```python
from build123d import *

# Parameters (mm, degrees)
SKETCH1_R           = 10.5
BOSS_EXTRUDE1_DEPTH = 10
SKETCH2_W           = 10.583005244
SKETCH2_H           = 12
BOSS_EXTRUDE2_DEPTH = 16
CUT_EXTRUDE1_REACH  = 34.181
SKETCH3_R           = 3
SKETCH4_R           = 8.7
BOSS_EXTRUDE3_DEPTH = 242
BOSS_EXTRUDE4_START = 10
SKETCH5_R           = 10.5
BOSS_EXTRUDE4_DEPTH = 10
BOSS_EXTRUDE5_START = 17
SKETCH6_R           = 8
BOSS_EXTRUDE5_DEPTH = 17
SKETCH7_R           = 3
CUT_EXTRUDE2_DEPTH  = 201


with BuildPart() as part:
    # Sketch1 → Boss-Extrude1 (new body)
    with BuildSketch(Plane.XY):
        Circle(SKETCH1_R)
    extrude(amount=BOSS_EXTRUDE1_DEPTH)

    # Sketch2 → Boss-Extrude2 (add)
    with BuildSketch(Plane.XY.offset(10)):
        Rectangle(SKETCH2_W, SKETCH2_H)
        with BuildLine():
            ThreePointArc((5.291502622, 6), (0, 8), (-5.291502622, 6))
            Line((-5.291502622, 6), (5.291502622, 6))
        make_face()
        with BuildLine():
            Line((5.291502622, -6), (-5.291502622, -6))
            ThreePointArc((-5.291502622, -6), (0, -8), (5.291502622, -6))
        make_face()
    extrude(amount=BOSS_EXTRUDE2_DEPTH)

    # Sketch3 → Cut-Extrude1 (cut, up to next)
    with BuildSketch(Plane(origin=(5.291502622, 0, 0), x_dir=(0, 0, -1), z_dir=(1, 0, 0)), mode=Mode.PRIVATE) as cut_extrude1_sk1:
        with Locations((-19, 0)):
            Circle(SKETCH3_R)
    cut_extrude1_tool1 = extrude(cut_extrude1_sk1.sketch, amount=-CUT_EXTRUDE1_REACH, mode=Mode.PRIVATE) & part.part
    add(cut_extrude1_tool1.solids().sort_by_distance((5.291503, 0, 19))[0], mode=Mode.SUBTRACT)

    # Sketch4 → Boss-Extrude3 (add)
    with BuildSketch(Plane(origin=(0, 0, 0), x_dir=(-1, 0, 0), z_dir=(0, 0, -1))):
        with Locations(Location((0, 0, 0), (0, 0, 180))):
            Circle(SKETCH4_R)
    extrude(amount=BOSS_EXTRUDE3_DEPTH)

    # Sketch5 → Boss-Extrude4 (add)
    with BuildSketch(Plane(origin=(0, 0, -242), x_dir=(-1, 0, 0), z_dir=(0, 0, -1)).offset(BOSS_EXTRUDE4_START)):
        with Locations(Location((0, 0, 0), (0, 0, 180))):
            Circle(SKETCH5_R)
    extrude(amount=-BOSS_EXTRUDE4_DEPTH)

    # Sketch6 → Boss-Extrude5 (add)
    with BuildSketch(Plane(origin=(0, 0, -252), x_dir=(-1, 0, 0), z_dir=(0, 0, -1)).offset(BOSS_EXTRUDE5_START)):
        Circle(SKETCH6_R)
    extrude(amount=-BOSS_EXTRUDE5_DEPTH)

    # Sketch7 → Cut-Extrude2 (cut)
    with BuildSketch(Plane(origin=(0, 0, -269), x_dir=(-1, 0, 0), z_dir=(0, 0, -1))):
        Circle(SKETCH7_R)
    extrude(amount=-CUT_EXTRUDE2_DEPTH, mode=Mode.SUBTRACT)


solid = part.part
```
Check sheet for the modelled part. Datum: model origin and axes. Units: mm. A direction names the side the tool comes from. Give positions to 0.01 mm unless a question says otherwise; leave off trailing zeros. Order: outer loops, then holes, each group sorted by start corner. A loop starts at its lowest first (then second) coordinate and runs counter-clockwise, first axis right, second up. Notation, with made-up numbers: M 33,21.5 L 72,21.5 A31 cw 72,57.5 Z; hole C -36.75,87 d3. An arc over 180 degrees is marked long. Answer in a Markdown table with one row per item.
1) Thickness scan on L1, parallel to Y at x = 0, z = -216.5; L2, parallel to Z at x = -8, y = -6.75; L3, parallel to Z at x = 2, y = -0.25. Record the ranges inside material, lowest first. Write a range as [from, to].
Filled sheet:
| item | result |
|---|---|
| L1 | y = [-8.7, -3], [3, 8.7] |
| L2 | z = [-252, -242], [0, 10] |
| L3 | z = [-68, 16.01], [21.99, 26] |
2) Gauge pin test, flat ends, axial feed: P1, Ø1.5, axis at x = 5.5, z = -48.5, coming from the +Y side; P2, Ø12, axis at x = 5, z = -136.5, coming from the -Y side; P3, Ø3.5, axis at y = -1, z = 17, coming from the +X side; P4, Ø10, axis at x = 6, y = 1, coming from the +Z side. Record the tip position at first contact, or that the pin passes through.
Filled sheet:
| item | result |
|---|---|
| P1 | stops at y = 7.29 |
| P2 | stops at y = -8.7 |
| P3 | stops at x = 5.29 |
| P4 | stops at z = 26 |
3) Access from +Z, -Z, +X, -X, +Y, -Y to the whole of each face (thin tool, end or side, straight path). Record for faces 5 (the flat face through (-2, 8, -252)), 6 (the flat face through (7, 0, 10)), 7 (the cylindrical face through (-1.886, 8.493, -119.306)), 8 (the cylindrical face through (0, 8, 18)).
Filled sheet:
| item | result |
|---|---|
| face 5 | -Z |
| face 6 | +Z |
| face 7 | none |
| face 8 | +Z, +Y |
4) Cross-section at B-B, the plane x = 0. Enter the section's corners in (y, z).
Filled sheet:
| item | result |
|---|---|
| outline | M -10.5,-252 L -8,-252 L -8,-269 L -3,-269 L -3,-68 L 3,-68 L 3,-269 L 8,-269 L 8,-252 L 10.5,-252 L 10.5,-242 L 8.7,-242 L 8.7,0 L 10.5,0 L 10.5,10 L 8,10 L 8,26 L -8,26 L -8,10 L -10.5,10 L -10.5,0 L -8.7,0 L -8.7,-242 L -10.5,-242 Z; hole C 0,19 d6 |
5) Cross-section at D-D, the plane z = -156. Enter the section's corners in (x, y).
Filled sheet:
| item | result |
|---|---|
| outline | C 0,0 d17.4; hole C 0,0 d6 |
6) Cross-section at A-A, the plane y = 0. Enter the section's corners in (x, z), plus the area to 3 significant figures.
Filled sheet:
| item | result |
|---|---|
| outline | M -10.5,-252 L -8,-252 L -8,-269 L -3,-269 L -3,-68 L 3,-68 L 3,-269 L 8,-269 L 8,-252 L 10.5,-252 L 10.5,-242 L 8.7,-242 L 8.7,0 L 10.5,0 L 10.5,10 L 5.29,10 L 5.29,16 L -5.29,16 L -5.29,10 L -10.5,10 L -10.5,0 L -8.7,0 L -8.7,-242 L -10.5,-242 Z; M -5.29,22 L 5.29,22 L 5.29,26 L -5.29,26 Z |
| area | 3,800 mm2 |
7) Cross-section at C-C, the plane z = 19. Enter the section's corners in (x, y).
Filled sheet:
| item | result |
|---|---|
| outline | M -5.29,-6 A8 ccw 5.29,-6 L 5.29,-3 L -5.29,-3 Z; M -5.29,3 L 5.29,3 L 5.29,6 A8 ccw -5.29,6 Z |
8) Release check for a two-part mould opening along Z. For faces 1 (the flat face through (-5.292, -1, 16)), 2 (the flat face through (0, 0, 26)), 3 (the flat face through (-4, -8, -242)), 4 (the flat face through (0, 0, -68)) record: +Z half, -Z half, draft (parallel to the pull), parting line (faces both ways), or undercut.
Filled sheet:
| item | result |
|---|---|
| face 1 | draft |
| face 2 | +Z half |
| face 3 | undercut |
| face 4 | -Z half |
